Input: part model. Units: mm. Frame: model coordinates. Coordinates: 2 decimals unless noted, no trailing zeros. Write each loop counter-clockwise with the first axis right and the second up, starting at its lowest first coordinate (ties: lowest second). Pieces come first, ordered by that corner, then holes. Notation, with made-up numbers: M 31,-13 L 75,-13 A27 ccw 75,11 Z; hole C 74,43.25 d2. An arc over 180 degrees is marked long. Answer as a JSON object with one key per item and string values. Group by question number.
from build123d import *

# Parameters (mm, degrees)
BOSS_EXTRUDE1_DEPTH = 5
SKETCH5_R           = 5
CUT_EXTRUDE2_DEPTH  = 10


with BuildPart() as part:
    # Sketch1 → Boss-Extrude1 (new body)
    with BuildSketch(Plane(origin=(0, 0, 0), x_dir=(1, 0, 0), z_dir=(0, 1, 0))):
        with BuildLine():
            ThreePointArc((-89.202352286, -85), (-81.880021816, -102.67766953), (-64.202352286, -110))
            Line((-64.202352286, -110), (65.797647714, -110))
            ThreePointArc((65.797647714, -110), (83.475317244, -102.67766953), (90.797647714, -85))
            Line((90.797647714, -85), (90.797647714, -35))
            Line((90.797647714, -35), (90.797647714, 31.47331922))
            Line((90.797647714, 31.47331922), (90.797647714, 79.461679372))
            ThreePointArc((90.797647714, 79.461679372), (84.910138891, 95.577283021), (70.020633234, 104.102425978))
            ThreePointArc((70.020633234, 104.102425978), (0.80038099, 109.994179998), (-68.420925207, 104.11482166))
            ThreePointArc((-68.420925207, 104.11482166), (-83.313400439, 95.590634086), (-89.202352286, 79.47331922))
            Line((-89.202352286, 79.47331922), (-89.202352286, 31.47331922))
            Line((-89.202352286, 31.47331922), (-89.202352286, -35))
            Line((-89.202352286, -35), (-89.202352286, -85))
        make_face()
    extrude(amount=BOSS_EXTRUDE1_DEPTH)

    # Sketch5 → Cut-Extrude2 (cut)
    with BuildSketch(Plane(origin=(0, 5, 0), x_dir=(1, 0, 0), z_dir=(0, 1, 0))):
        with Locations((-77.202352286, 20)):
            Circle(SKETCH5_R)
        with Locations((-77.202352286, -20)):
            Circle(SKETCH5_R)
        with Locations((-77.202352286, 87.5)):
            Circle(SKETCH5_R)
        with Locations((-77.202352286, -94)):
            Circle(SKETCH5_R)
        Circle(SKETCH5_R)
        with Locations((77.202352286, -94)):
            Circle(SKETCH5_R)
        with Locations((77.202352286, -20)):
            Circle(SKETCH5_R)
        with Locations((77.202352286, 20)):
            Circle(SKETCH5_R)
        with Locations((77.202352286, 87.5)):
            Circle(SKETCH5_R)
    extrude(amount=-CUT_EXTRUDE2_DEPTH, mode=Mode.SUBTRACT)


solid = part.part
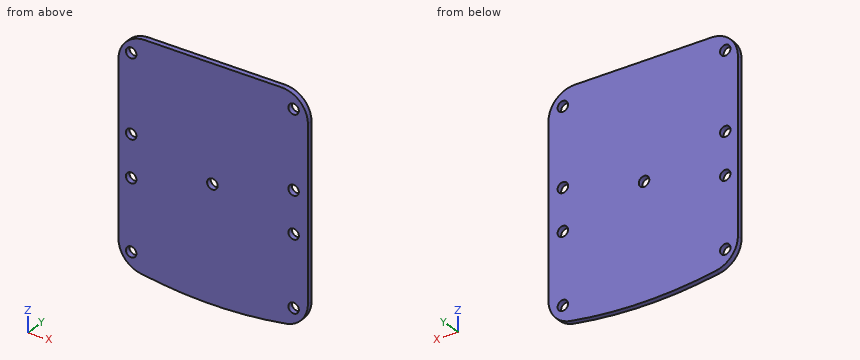
Q1. Section C-C, the plane y = 3.7. State how many separate pieces and enclosed holes the cut face has, and give its area (3 significant figures).
Q2. Section B-B, the plane z = -20. Return the cut outline in (x, y), and give its area (3 significant figures).
Q3. Section D-D, the plane z = -87.5. Return the cut outline in (x, y), and give its area (3 significant figures).
Q4. Line query: line 1 (X direction, y = 2.2, z = 20); line 2 (X direction, y = 2.4, z = 0); line 3 (X direction, y = 2, z = -22). Output: solid intervals per line, ascending. Write a range as from..to.
Q5. Section A-A, the plane x = 0. Return the cut outline in (y, z), and give its area (3 significant figures).
Filled in:
{
 "1": {"separate pieces": "1", "enclosed holes": "9", "area": "37,900 mm^2"},
 "2": {"outline": "M -89.2,0 L -82.2,0 L -82.2,5 L -89.2,5 Z; M -72.2,0 L 72.2,0 L 72.2,5 L -72.2,5 Z; M 82.2,0 L 90.8,0 L 90.8,5 L 82.2,5 Z", "area": "800 mm^2"},
 "3": {"outline": "M -87.88,0 L -82.2,0 L -82.2,5 L -87.88,5 Z; M -72.2,0 L 72.2,0 L 72.2,5 L -72.2,5 Z; M 82.2,0 L 89.47,0 L 89.47,5 L 82.2,5 Z", "area": "787 mm^2"},
 "4": {"line 1": "-89.2..-82.2, -72.2..72.2, 82.2..90.8", "line 2": "-89.2..-5, 5..90.8", "line 3": "-89.2..-81.78, -72.62..72.62, 81.78..90.8"},
 "5": {"outline": "M 0,-109.99 L 5,-109.99 L 5,-5 L 0,-5 Z; M 0,5 L 5,5 L 5,110 L 0,110 Z", "area": "1,050 mm^2"}
}
